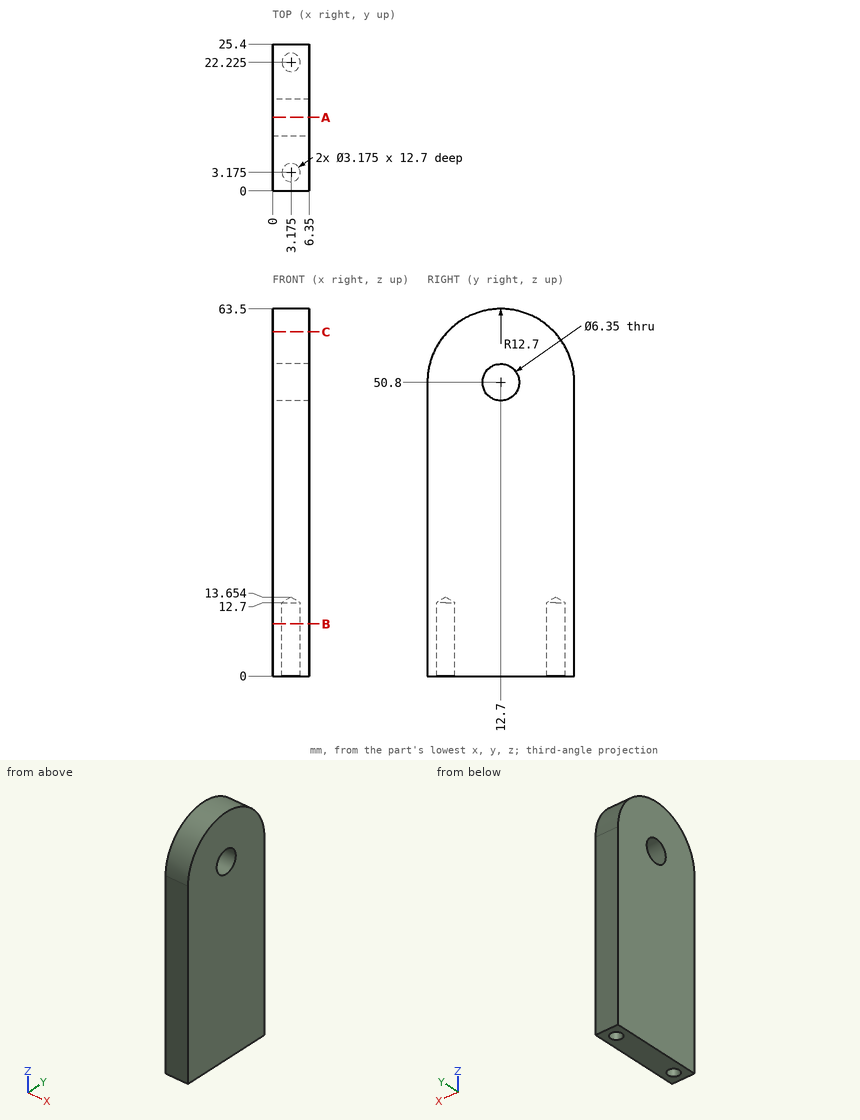
Here's the drawing with two shaded views (mm, measured from the low corner). I have some questions. Coordinates: 2 decimals unless noted, no trailing zeros. Write each loop counter-clockwise with the first axis right and the second up, starting at its lowest first coordinate (ties: lowest second). Pieces come first, ordered by that corner, then holes. Notation, with made-up numbers: M -32,57 L 4,57 A28 cw 4,84 Z; hole C 67.5,25 d8. An arc over 180 degrees is marked long. Use one line per item in the form item = value.
Q1. If we section it at C-C (z = 59.5): Write out the boundary of the cut face in (x, y), then the cut area to 4 significant figures.
Model answer:
outline = M 0,3.45 L 6.35,3.45 L 6.35,21.95 L 0,21.95 Z
area = 117.5 mm^2
Q2. I need wall thicknesses on line 1 along Z through (x, y) = (1.5, 12.7) (3 decimals); line 2 along Y through (x, z) = (2.5, 3); line 3 along Y through (x, z) = (5.5, 49.5). Which ranges of each line are inside material? Lowest first, please. Write a range as from..to.
Model answer:
line_1 = 0..47.625, 53.975..63.5
line_2 = 0..1.74, 4.61..20.79, 23.66..25.4
line_3 = 0..9.8, 15.6..25.4
Q3. If we section it at B-B (z = 9): State how many separate pieces and enclosed holes the cut face has, then the cut area to 3 significant figures.
Model answer:
separate_pieces = 1
enclosed_holes = 2
area = 145 mm^2
Q4. If we section it at A-A (y = 12.7): Write out the boundary of the cut face in (x, z) (3 decimals).
Model answer:
outline = M 0,0 L 6.35,0 L 6.35,47.625 L 0,47.625 Z; M 0,53.975 L 6.35,53.975 L 6.35,63.5 L 0,63.5 Z
Q5. For P1, Ø3, axis at x = 3.5, y = 9, coming from the +Z side; P2, Ø2.5, axis at x = 3.175, y = 22.225, coming from the +Z side; P3, Ø1, axis at x = 5.5, z = 55.5, coming from the -Y side, each with a flat end and sliding along its axis, tell me the tip position at first contact or that it passes through.
Model answer:
P1 = 63.31
P2 = 60.43
P3 = 0.71
